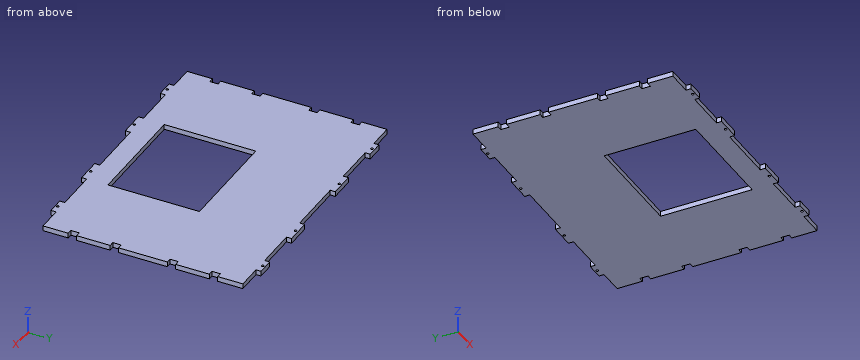
```python
from build123d import *

# Parameters (mm, degrees)
ESQUISSE1_W             = 330
ESQUISSE1_H             = 238
BOSS_EXTRU_1_DEPTH      = 6
ESQUISSE2_W             = 129
ESQUISSE2_H             = 109
ENL_V_MAT_EXTRU_1_DEPTH = 6
ESQUISSE3_W             = 20
ESQUISSE3_H             = 6
ESQUISSE3_W_2           = 30
BOSS_EXTRU_4_DEPTH      = 6
ESQUISSE4_W             = 6
ESQUISSE4_H             = 10
ENL_V_MAT_EXTRU_3_DEPTH = 6
ESQUISSE5_R             = 1.4
ENL_V_MAT_EXTRU_4_DEPTH = 6


with BuildPart() as part:
    # Esquisse1 → Boss.-Extru.1 (new body)
    with BuildSketch(Plane.XY):
        Rectangle(ESQUISSE1_W, ESQUISSE1_H)
    extrude(amount=BOSS_EXTRU_1_DEPTH)

    # Esquisse2 → Enlèv. mat.-Extru.1 (cut)
    with BuildSketch(Plane.XY.offset(6)):
        with Locations((0, -39.5)):
            Rectangle(ESQUISSE2_W, ESQUISSE2_H)
    extrude(amount=-ENL_V_MAT_EXTRU_1_DEPTH, mode=Mode.SUBTRACT)

    # Esquisse3 → Boss.-Extru.4 (add)
    with BuildSketch(Plane.XY.offset(6)):
        with Locations((-125, 122)):
            Rectangle(ESQUISSE3_W, ESQUISSE3_H)
        with Locations((-50, 122)):
            Rectangle(ESQUISSE3_W_2, ESQUISSE3_H)
        with Locations((50, 122)):
            Rectangle(ESQUISSE3_W_2, ESQUISSE3_H)
        with Locations((125, 122)):
            Rectangle(ESQUISSE3_W, ESQUISSE3_H)
        with Locations((125, -122)):
            Rectangle(ESQUISSE3_W, ESQUISSE3_H)
        with Locations((50, -122)):
            Rectangle(ESQUISSE3_W_2, ESQUISSE3_H)
        with Locations((-50, -122)):
            Rectangle(ESQUISSE3_W_2, ESQUISSE3_H)
        with Locations((-125, -122)):
            Rectangle(ESQUISSE3_W, ESQUISSE3_H)
    extrude(amount=-BOSS_EXTRU_4_DEPTH)

    # Esquisse4 → Enlèv. mat.-Extru.3 (cut)
    with BuildSketch(Plane.XY.offset(6)):
        with Locations((-162, 84)):
            Rectangle(ESQUISSE4_W, ESQUISSE4_H)
        with Locations((-162, 34)):
            Rectangle(ESQUISSE4_W, ESQUISSE4_H)
        with Locations((-162, -84)):
            Rectangle(ESQUISSE4_W, ESQUISSE4_H)
        with Locations((-162, -34)):
            Rectangle(ESQUISSE4_W, ESQUISSE4_H)
        with Locations((162, -84)):
            Rectangle(ESQUISSE4_W, ESQUISSE4_H)
        with Locations((162, -34)):
            Rectangle(ESQUISSE4_W, ESQUISSE4_H)
        with Locations((162, 34)):
            Rectangle(ESQUISSE4_W, ESQUISSE4_H)
        with Locations((162, 84)):
            Rectangle(ESQUISSE4_W, ESQUISSE4_H)
    extrude(amount=-ENL_V_MAT_EXTRU_3_DEPTH, mode=Mode.SUBTRACT)

    # Esquisse5 → Enlèv. mat.-Extru.4 (cut)
    with BuildSketch(Plane.XY.offset(6)):
        with Locations((-125, 122)):
            Circle(ESQUISSE5_R)
        with Locations((-50, 122)):
            Circle(ESQUISSE5_R)
        with Locations((50, 122)):
            Circle(ESQUISSE5_R)
        with Locations((125, 122)):
            Circle(ESQUISSE5_R)
        with Locations((125, -122)):
            Circle(ESQUISSE5_R)
        with Locations((50, -122)):
            Circle(ESQUISSE5_R)
        with Locations((-50, -122)):
            Circle(ESQUISSE5_R)
        with Locations((-125, -122)):
            Circle(ESQUISSE5_R)
    extrude(amount=-ENL_V_MAT_EXTRU_4_DEPTH, mode=Mode.SUBTRACT)


solid = part.part
```
The model under review builds one solid part; all positions refer to its coordinate system, in mm. Round coordinates to 2 decimals unless told otherwise and drop trailing zeros. Loops run counter-clockwise (first coordinate to the right, second up) from the corner with the lowest first, then second, coordinate; pieces in that order, holes last. Notation, with made-up numbers: (84.5, 2.5) -> (121.5, 2.5) arc R15 cw to (121.5, 28.5) -> close; hole circle Ø8 at (26, 11). An arc over 180 degrees is marked (long way). Answer in a Markdown table with one row per item.
1) For pin 1 Ø2 at (y, z) = (32.5, 2.5) entering from +X; pin 2 Ø1.8 at (x, z) = (-155.5, 1.5) entering from -Y; pin 3 Ø3 at (x, z) = (-161.5, 3.5) entering from +Y; pin 4 Ø2 at (x, y) = (-125, 122) entering from +Z, all flat-tipped, find the tip position at first contact; note any pin that passes through.
Taken from the geometry:
| item | result |
|---|---|
| pin 1 | stops at x = 159 |
| pin 2 | stops at y = -119 |
| pin 3 | stops at y = 119 |
| pin 4 | passes through |
2) Consider section D-D, the plane x = 99.5. Write out the cut boundary in (y, z), plus the area to 3 significant figures.
Taken from the geometry:
| item | result |
|---|---|
| outline | (-119, 0) -> (119, 0) -> (119, 6) -> (-119, 6) -> close |
| area | 1,430 mm² |
3) Consider section C-C, the plane x = -21.5. Write out the cut boundary in (y, z), plus the area to 3 significant figures.
Taken from the geometry:
| item | result |
|---|---|
| outline | (-119, 0) -> (-94, 0) -> (-94, 6) -> (-119, 6) -> close; (15, 0) -> (119, 0) -> (119, 6) -> (15, 6) -> close |
| area | 774 mm² |
4) Consider section B-B, the plane z = 3.7. Count the separate pieces of the cut face and the enclosed holes in it, plus the area to 3 significant figures.
Taken from the geometry:
| item | result |
|---|---|
| separate pieces | 1 |
| enclosed holes | 9 |
| area | 65,100 mm² |
5) Wall thickness on line 1 along Y through (x, z) = (125, 3.9); line 2 along Y through (x, z) = (-50, 3.6); line 3 along X through (y, z) = (-77, 0.95): over which ranges is each line inside the solid? List them lowest first.
Taken from the geometry:
| item | result |
|---|---|
| line 1 | y = -125 to -123.4, -120.6 to 120.6, 123.4 to 125 |
| line 2 | y = -125 to -123.4, -120.6 to -94, 15 to 120.6, 123.4 to 125 |
| line 3 | x = -165 to -64.5, 64.5 to 165 |
6) Consider section A-A, the plane x = 42.5. Write out the cut boundary in (y, z), plus the area to 3 significant figures.
Taken from the geometry:
| item | result |
|---|---|
| outline | (-125, 0) -> (-94, 0) -> (-94, 6) -> (-125, 6) -> close; (15, 0) -> (125, 0) -> (125, 6) -> (15, 6) -> close |
| area | 846 mm² |
